Source: CAD feature listing. Evaluate the final solid. Frame: model axes, mm. Face numbers are marked on the shaded views. A direction names the side the tool comes from. Coordinates: 2 decimals unless noted, no trailing zeros. Order: outer loops, then holes, each group sorted by start corner. A loop starts at its lowest first (then second) coordinate and runs counter-clockwise, first axis right, second up. Notation, with made-up numbers: (-3.75, 9) - (35.25, 9) arc R25 cw to (35.25, 44) - close; hole circle Ø1 at (43, 35). An arc over 180 degrees is marked (long way). One line per question, with ' | ' between items.
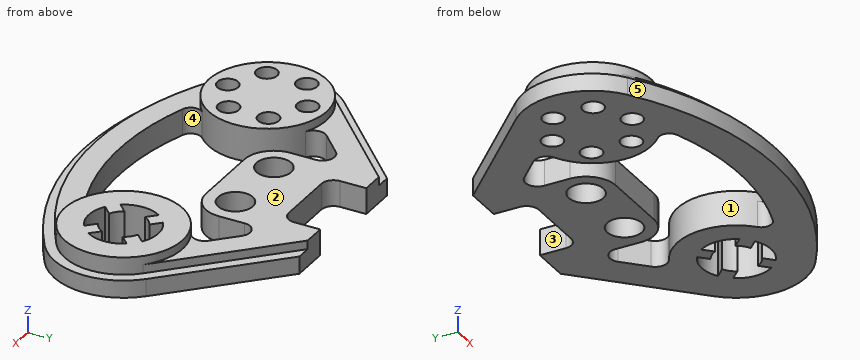
from build123d import *

# Parameters (mm, degrees)
EXTRUDE_1_DEPTH = 10
SKETCH_1_3_R    = 34
SKETCH_1_3_R_2  = 6
EXTRUDE_2_DEPTH = 20
SKETCH_1_4_R    = 10
EXTRUDE_3_DEPTH = 15


with BuildPart() as part:
    # Sketch 1 → Extrude 1 (new body)
    with BuildSketch(Plane.XY):
        with BuildLine():
            Line((120.561139783, 85), (112, 85))
            Line((112, 85), (173.82860287, 24.252787165))
            ThreePointArc((173.82860287, 24.252787165), (181.354206237, 13.149667342), (184, 0))
            ThreePointArc((184, 0), (180.106628687, -15.798446414), (169.318181818, -27.97870353))
            ThreePointArc((169.318181818, -27.97870353), (75, -57.376798059), (-19.318181818, -27.97870353))
            ThreePointArc((-19.318181818, -27.97870353), (-33.873934113, -2.92516456), (-23.82860287, 24.252787165))
            Line((-23.82860287, 24.252787165), (38, 85))
            Line((38, 85), (29.438860217, 85))
            Line((29.438860217, 85), (-28.033650435, 28.532690783))
            ThreePointArc((-28.033650435, 28.532690783), (-39.851687192, -3.441370071), (-22.727272727, -32.9161218))
            ThreePointArc((-22.727272727, -32.9161218), (75, -63.376798059), (172.727272727, -32.9161218))
            ThreePointArc((172.727272727, -32.9161218), (189.851687192, -3.441370071), (178.033650435, 28.532690783))
            Line((178.033650435, 28.532690783), (120.561139783, 85))
        make_face()
    extrude(amount=EXTRUDE_1_DEPTH)

    # Sketch 1_3 → Extrude 2 (add)
    # profile 1 of 2: a face of its own
    with BuildSketch(Plane.XY):
        with Locations(Location((0, 0, 0), (0, 0, 134.494537505))):
            Circle(SKETCH_1_3_R)
        with Locations((-19.918584287, 11.5)):
            Circle(SKETCH_1_3_R_2, mode=Mode.SUBTRACT)
        with Locations((-19.918584287, -11.5)):
            Circle(SKETCH_1_3_R_2, mode=Mode.SUBTRACT)
        with Locations((0, -23)):
            Circle(SKETCH_1_3_R_2, mode=Mode.SUBTRACT)
        with Locations((19.918584287, -11.5)):
            Circle(SKETCH_1_3_R_2, mode=Mode.SUBTRACT)
        with Locations((19.918584287, 11.5)):
            Circle(SKETCH_1_3_R_2, mode=Mode.SUBTRACT)
        with Locations((0, 23)):
            Circle(SKETCH_1_3_R_2, mode=Mode.SUBTRACT)
    # profile 2 of 2: a face of its own
    with BuildSketch(Plane.XY):
        with Locations(Location((150, 0, 0), (0, 0, 304.623535479))):
            Circle(SKETCH_1_3_R)
        with BuildLine():
            ThreePointArc((161.027979336, 16.684833585), (150, 20), (138.972020664, 16.684833585))
            Line((138.972020664, 16.684833585), (144.081999282, 11.574854967))
            ThreePointArc((144.081999282, 11.574854967), (140.807611845, 9.192388155), (138.425145033, 5.918000718))
            Line((138.425145033, 5.918000718), (133.315166415, 11.027979336))
            ThreePointArc((133.315166415, 11.027979336), (130, 0), (133.315166415, -11.027979336))
            Line((133.315166415, -11.027979336), (138.425145033, -5.918000718))
            ThreePointArc((138.425145033, -5.918000718), (140.807611845, -9.192388155), (144.081999282, -11.574854967))
            Line((144.081999282, -11.574854967), (138.972020664, -16.684833585))
            ThreePointArc((138.972020664, -16.684833585), (150, -20), (161.027979336, -16.684833585))
            Line((161.027979336, -16.684833585), (155.918000718, -11.574854967))
            ThreePointArc((155.918000718, -11.574854967), (159.192388155, -9.192388155), (161.574854967, -5.918000718))
            Line((161.574854967, -5.918000718), (166.684833585, -11.027979336))
            ThreePointArc((166.684833585, -11.027979336), (170, 0), (166.684833585, 11.027979336))
            Line((166.684833585, 11.027979336), (161.574854967, 5.918000718))
            ThreePointArc((161.574854967, 5.918000718), (159.192388155, 9.192388155), (155.918000718, 11.574854967))
            Line((155.918000718, 11.574854967), (161.027979336, 16.684833585))
        make_face(mode=Mode.SUBTRACT)
    extrude(amount=EXTRUDE_2_DEPTH)

    # Sketch 1_4 → Extrude 3 (add)
    # profile 1 of 2: a face of its own
    with BuildSketch(Plane.XY):
        with BuildLine():
            Line((173.82860287, 24.252787165), (112, 85))
            Line((112, 85), (99, 85))
            Line((99, 85), (99, 70))
            ThreePointArc((99, 70), (96.949747468, 65.050252532), (92, 63))
            Line((92, 63), (58, 63))
            ThreePointArc((58, 63), (53.050252532, 65.050252532), (51, 70))
            Line((51, 70), (51, 85))
            Line((51, 85), (38, 85))
            Line((38, 85), (-23.82860287, 24.252787165))
            ThreePointArc((-23.82860287, 24.252787165), (-5.164889991, 33.605414912), (15.445958822, 30.28898077))
            ThreePointArc((15.445958822, 30.28898077), (11.707247274, 35.461587695), (13.720120341, 41.518168286))
            Line((13.720120341, 41.518168286), (26.094111174, 53.675736464))
            ThreePointArc((26.094111174, 53.675736464), (33.707284453, 55.137793332), (38, 48.682515577))
            Line((38, 48.682515577), (38, 34))
            ThreePointArc((38, 34), (42.97918472, 21.97918472), (55, 17))
            Line((55, 17), (95, 17))
            ThreePointArc((95, 17), (107.02081528, 21.97918472), (112, 34))
            Line((112, 34), (112, 48.682515577))
            ThreePointArc((112, 48.682515577), (116.292715547, 55.137793332), (123.905888826, 53.675736464))
            Line((123.905888826, 53.675736464), (136.279879659, 41.518168286))
            ThreePointArc((136.279879659, 41.518168286), (138.292752726, 35.461587695), (134.554041178, 30.28898077))
            ThreePointArc((134.554041178, 30.28898077), (155.164889991, 33.605414912), (173.82860287, 24.252787165))
        make_face()
        with Locations((55, 34)):
            Circle(SKETCH_1_4_R, mode=Mode.SUBTRACT)
        with Locations((95, 34)):
            Circle(SKETCH_1_4_R, mode=Mode.SUBTRACT)
    # profile 2 of 2: a face of its own
    with BuildSketch(Plane.XY):
        with BuildLine():
            ThreePointArc((-19.318181818, -27.97870353), (75, -57.376798059), (169.318181818, -27.97870353))
            ThreePointArc((169.318181818, -27.97870353), (147.563945827, -33.912617712), (126.881190396, -24.930315732))
            ThreePointArc((126.881190396, -24.930315732), (128.673214982, -30.563393481), (124.765841582, -34.999083974))
            ThreePointArc((124.765841582, -34.999083974), (75, -43.376798059), (25.234158418, -34.999083974))
            ThreePointArc((25.234158418, -34.999083974), (21.326785018, -30.563393481), (23.118809604, -24.930315732))
            ThreePointArc((23.118809604, -24.930315732), (2.436054173, -33.912617712), (-19.318181818, -27.97870353))
        make_face()
    extrude(amount=EXTRUDE_3_DEPTH)


solid = part.part
(1) Cut plane D-D (x = -1). Return the cut outline in (y, z).
Taken from the geometry:
outline: (-45.68, 0) - (-28.92, 0) - (-28.92, 20) - (-33.99, 20) - (-33.99, 15) - (-38.96, 15) - (-38.96, 10) - (-45.68, 10) - close; (-17.08, 0) - (17.08, 0) - (17.08, 20) - (-17.08, 20) - close; (28.92, 0) - (55.09, 0) - (55.09, 10) - (46.68, 10) - (46.68, 15) - (33.99, 15) - (33.99, 20) - (28.92, 20) - close
(2) Set-up query: the marked faces 1, 2, 3, 4 and 5. Return all of +Z, -Z, +X, -X, +Y, -Y with unobstructed straight access to the full face (end or side cutting, diameter ignored); none if empty.
Taken from the geometry:
face 1: +Z | face 2: +Z, +Y | face 3: +Z, -Z, +Y | face 4: +Z, -Z | face 5: +Z, -Z, -Y
(3) Cut plane B-B (z = 17.25). State how many separate pieces and enclosed holes the cut face has, and give its area (3 significant figures).
Taken from the geometry:
separate pieces: 2 | enclosed holes: 7 | area: 5,550 mm²
(4) Pin query (flat end, axial travel): P1, Ø19, axis at x = 19.92, y = -11.5, coming from the -Z side; P2, Ø20.5, axis at x = 32, y = 36.5, coming from the +Z side; P3, Ø10, axis at y = 39, z = 7.5, coming from the +X side; P4, Ø8, axis at y = -36.5, z = 9, coming from the +X side. Return the tip coordinate at first contact, or that it passes through.
Taken from the geometry:
P1: stops at z = 0 | P2: stops at z = 15 | P3: stops at x = 172.47 | P4: stops at x = 173.32
(5) Cut plane A-A (y = 0). Return the cut outline in (x, z), and give its area (3 significant figures).
Taken from the geometry:
outline: (-40, 0) - (34, 0) - (34, 20) - (-34, 20) - (-34, 10) - (-40, 10) - close; (116, 0) - (130, 0) - (130, 20) - (116, 20) - close; (170, 0) - (190, 0) - (190, 10) - (184, 10) - (184, 20) - (170, 20) - close | area: 2,040 mm²
(6) Material intervals for L1, parallel to Y at x = 5.5, z = 5.5; L2, parallel to X at y = 38.5, z = 9.25; L3, parallel to X at y = -21.5, z = 1, sorted ascending. Write a range as from..to.
Taken from the geometry:
L1: y = -48.71..-25.4, -20.6..20.6, 25.4..61.48 | L2: x = -17.89..11.91, 38..46.07, 63.93..86.07, 103.93..112, 138.09..167.89 | L3: x = -33.73..-5.81, 5.81..26.34, 123.66..183.73
(7) Cut plane C-C (x = 75). Return the cut outline in (y, z).
Taken from the geometry:
outline: (-63.38, 0) - (-43.38, 0) - (-43.38, 15) - (-57.38, 15) - (-57.38, 10) - (-63.38, 10) - close; (17, 0) - (63, 0) - (63, 15) - (17, 15) - close
